Autodesk Inventor part; units mm, degrees
ref_plane "YZ Plane" through (0, 0, 0) normal (1, 0, 0) x (0, 1, 0)
ref_plane "XZ Plane" through (0, 0, 0) normal (0, 1, 0) x (-1, 0, 0)
ref_plane "XY Plane" through (0, 0, 0) normal (0, 0, 1) x (1, 0, 0)
sketch "Skizze1" plane through (0, 0, 0) normal (0, 0, 1) x (1, 0, 0)
  line L0 (-23.5, 19.5) -> (23.5, 19.5)
  line L1 (23.5, 19.5) -> (23.5, -19.5)
  line L2 (23.5, -19.5) -> (-23.5, -19.5)
  line L3 (-23.5, -19.5) -> (-23.5, 19.5)
  line L4 (-23.5, -19.5) -> (23.5, 19.5) construction
  circle A0 centre (-21.0614, 17.0614) radius 1
  circle A1 centre (16, 0) radius 1.5
  line L5 (-23.5, 0) -> (23.5, 0) construction
  circle A2 centre (-21.0614, -17.0614) radius 1
  line L6 (-21.0614, -17.0614) -> (-21.0614, 17.0614) construction
  line L7 (-23.5, 19.5) -> (-21.0614, 17.0614) construction
  line L8 (12.5, -18.5) -> (29.5, -18.5)
  line L9 (29.5, -18.5) -> (29.5, -3.3)
  line L10 (29.5, -3.3) -> (12.5, -3.3)
  line L11 (12.5, -3.3) -> (12.5, -18.5)
  line L12 (12.5, 3.3) -> (29.5, 3.3)
  line L13 (29.5, 3.3) -> (29.5, 18.5)
  line L14 (29.5, 18.5) -> (12.5, 18.5)
  line L15 (12.5, 18.5) -> (12.5, 3.3)
  circle A3 centre (-5.25, -13.5) radius 5
  circle A4 centre (5.25, -13.5) radius 5
  circle A5 centre (-5.25, 13.5) radius 5
  circle A6 centre (5.25, 13.5) radius 5
  circle A7 centre (0, 0) radius 8
  circle A8 centre (0, 0) radius 4
  line L16 (-23.4, 5.9386) -> (-11.75, 5.9386)
  line L17 (-11.75, 5.9386) -> (-11.75, 14.9386)
  line L18 (-11.75, 14.9386) -> (-23.4, 14.9386)
  line L19 (-23.4, 14.9386) -> (-23.4, 5.9386)
  line L20 (-23.4, -15.0614) -> (-16.4, -15.0614)
  line L21 (-16.4, -15.0614) -> (-16.4, 4.9386)
  line L22 (-16.4, 4.9386) -> (-23.4, 4.9386)
  line L23 (-23.4, 4.9386) -> (-23.4, -15.0614)
  line L24 (0, 19.5) -> (0, -19.5) construction
  line L25 (-16.3, -18.5) -> (-10.5, -18.5)
  line L26 (-10.5, -18.5) -> (-10.5, 4.9386)
  line L27 (-10.5, 4.9386) -> (-16.3, 4.9386)
  line L28 (-16.3, 4.9386) -> (-16.3, -18.5)
  dimension "d0" = 39
  dimension "d1" = 47
  dimension "d2" = 3
  dimension "d3" = 2
  dimension "d4" = 38.3
  dimension "d5" = 6
  dimension "d6" = 45
  dimension "d7" = 10
  dimension "d8" = 0.5
  dimension "d9" = 1
  dimension "d10" = 16
  dimension "d11" = 15.2
  dimension "d13" = 6
  dimension "d14" = 17
  dimension "d15" = 15.2
  dimension "d16" = 1
  dimension "d17" = 8
  dimension "d18" = 20
  dimension "d19" = 7
  dimension "d20" = 0.1
  dimension "d21" = 5.8
  dimension "d22" = 0.1
  dimension "d23" = 1
  dimension "d24" = 1
  dimension "d25" = 0.1
  dimension "d26" = 9
  dimension "d27" = 1
  dimension "d28" = 1.5
extrude "Extrusion1" add sketch "Skizze1" against normal blind 2.2 contours L0 L1 L14 L15 L12 L10 L11 L8 L2 L3 | L1 L12 L15 L14 | L8 L11 L10 L1 | A3 | A4 | A5 | A6 | A7 | A8 | L19 L18 L17 L16 | L23 L22 L21 L20 | L28 L27 L26 L25
extrude "Extrusion2" add sketch "Skizze1" along normal blind 16.2 contours L14 L13 L12 L1 | L1 L12 L15 L14 | L8 L11 L10 L1 | L1 L10 L9 L8
sketch "Skizze2" plane through (29.5, -18.5, 0) normal (1, 0, 0) x (0, 0, -1)
  line L0 (-14.8, 1.2) -> (-9.5, 1.2)
  line L1 (-9.5, 1.2) -> (-9.5, 14)
  line L2 (-9.5, 14) -> (-14.8, 14)
  line L3 (-14.8, 14) -> (-14.8, 1.2)
  line L4 (-6.4, 1.2) -> (-1.1, 1.2)
  line L5 (-1.1, 1.2) -> (-1.1, 14)
  line L6 (-1.1, 14) -> (-6.4, 14)
  line L7 (-6.4, 14) -> (-6.4, 1.2)
  line L8 (0, 0) -> (0, 15.2)
  line L9 (-16.2, 15.2) -> (-16.2, 0)
  line L10 (-16.2, 7.6) -> (0, 7.6) construction
  line L11 (0, 38) -> (0, -1)
  point P0 (0, 18.5)
  dimension "d33" = 1.1
  dimension "d34" = 5.3
  dimension "d35" = 5.3
  dimension "d36" = 3.1
  dimension "d37" = 12.8
extrude "Extrusion3" cut sketch "Skizze2" against normal blind 10
extrude "Extrusion4" add sketch "Skizze1" along normal blind 9.5 contours A3 | A4
mirror "Spiegeln1" about plane through (0, 0, 0) normal (0, 1, 0) of "Extrusion4", "Extrusion3"
extrude "Extrusion5" add sketch "Skizze1" along normal blind 13 contours A7
extrude "Extrusion6" add sketch "Skizze1" along normal blind 8 contours L23 L22 L21 L20
extrude "Extrusion11" add sketch "Skizze1" along normal blind 8 contours L19 L18 L17 L16
extrude "Extrusion7" add sketch "Skizze1" along normal blind 7 contours L28 L27 L26 L25
sketch "Skizze3" plane through (-16.3, -18.5, 0) normal (0, -1, 0) x (1, 0, 0)
  line L0 (0, 7) -> (5.8, 7)
  line L1 (0.8004, 7) -> (0.8004, 0.8568)
  line L2 (0.8004, 0.8568) -> (1.6289, 0.8568)
  line L3 (1.6289, 0.8568) -> (1.6289, 7)
  line L4 (2.4575, 7) -> (2.4575, 0.8568)
  line L5 (2.4575, 0.8568) -> (3.2861, 0.8568)
  line L6 (3.2861, 0.8568) -> (3.2861, 7)
  line L7 (4.1146, 7) -> (4.1146, 0.8568)
  line L8 (4.1146, 0.8568) -> (4.9432, 0.8568)
  line L9 (4.9432, 0.8568) -> (4.9432, 7)
  line L10 (0, 0) -> (0, 7)
  line L11 (5.8, 0) -> (5.8, 7)
  point P0 (16.3, 0)
  dimension "d48" = 5.8
  dimension "d49" = 0.8286
  dimension "d50" = 0.8286
  dimension "d51" = 0.8286
extrude "Extrusion8" cut sketch "Skizze3" against normal up to surface (23.4386 mm away)
fillet "Rundung1" radius 0.5 4 edges at (-10.25, -13.5, 9.5) (0.25, -13.5, 9.5) (-10.25, 13.5, 9.5) (0.25, 13.5, 9.5)
sketch "Skizze4" plane through (0, 0, 8) normal (0, 0, 1) x (1, 0, 0)
  circle A0 centre (-19.9, 2.1386) radius 1.6
  circle A1 centre (-19.9, -2.6614) radius 1.6
  circle A2 centre (-19.9, -7.4614) radius 1.6
  circle A3 centre (-19.9, -12.2614) radius 1.6
  line L0 (-16.4, 4.9386) -> (-23.4, 4.9386)
  line L1 (-19.9, 4.9386) -> (-19.9, -15.0614) construction
  line L2 (-16.4, -15.0614) -> (-23.4, -15.0614)
  line L3 (-23.4, -15.0614) -> (-23.4, 4.9386)
  line L4 (-23.4, -5.0614) -> (-16.4, -5.0614) construction
  point P0 (0, 0)
  dimension "d55" = 3.2
  dimension "d56" = 4.8
  dimension "d57" = 4.8
  dimension "d58" = 4.8
extrude "Extrusion9" cut sketch "Skizze4" against normal up to surface (8 mm away)
sketch "Skizze5" plane through (-23.4, -15.0614, 0) normal (-1, 0, 0) x (0, 0, 1)
  line L0 (0.5, 19.15) -> (5, 19.15)
  line L1 (5, 19.15) -> (5, 15.25)
  line L2 (5, 15.25) -> (0.5, 15.25)
  line L3 (0.5, 15.25) -> (0.5, 19.15)
  line L4 (0.5, 14.35) -> (5, 14.35)
  line L5 (5, 14.35) -> (5, 10.45)
  line L6 (5, 10.45) -> (0.5, 10.45)
  line L7 (0.5, 10.45) -> (0.5, 14.35)
  line L8 (0.5, 5.65) -> (5, 5.65)
  line L9 (5, 5.65) -> (5, 9.55)
  line L10 (5, 9.55) -> (0.5, 9.55)
  line L11 (0.5, 9.55) -> (0.5, 5.65)
  line L12 (0.5, 4.75) -> (5, 4.75)
  line L13 (5, 4.75) -> (5, 0.85)
  line L14 (5, 0.85) -> (0.5, 0.85)
  line L15 (0.5, 0.85) -> (0.5, 4.75)
  line L16 (8, 17.2) -> (5, 17.2) construction
  line L17 (0.5, 17.2) -> (5, 17.2) construction
  line L18 (0.5, 12.4) -> (5, 12.4) construction
  line L19 (8, 12.4) -> (5, 12.4) construction
  line L20 (8, 7.6) -> (5, 7.6) construction
  line L21 (0.5, 7.6) -> (5, 7.6) construction
  line L22 (8, 20) -> (8, 0) construction
  line L23 (0.5, 2.8) -> (5, 2.8) construction
  line L24 (5, 2.8) -> (8, 2.8) construction
  line L25 (0, 34.5614) -> (0, -4.4386) construction
  circle A0 centre (4, 25.5) radius 2.5
  line L26 (4, 30) -> (4, 21) construction
  line L27 (8, 25.5) -> (0, 25.5) construction
  line L28 (0, 30) -> (8, 30)
  line L29 (8, 30) -> (8, 21)
  line L30 (0, 21) -> (8, 21)
  line L31 (0, 21) -> (0, 30)
  point P0 (0, 15.0614)
  point P1 (4, 25.5)
  dimension "d61" = 0.5
  dimension "d62" = 4.5
  dimension "d63" = 3.9
  dimension "d66" = 5
extrude "Extrusion10" cut sketch "Skizze5" against normal blind 7 contours L0 L1 L2 L3 | L4 L5 L6 L7 | L11 L10 L9 L8 | L12 L13 L14 L15 | A0
equation "\"d15\" = d11"
properties part number "Step_Down_USB"
Check sheet for the modelled part. Datum: model origin and axes. Units: mm. A direction names the side the tool comes from. Give positions to 0.01 mm unless a question says otherwise; leave off trailing zeros. Write each loop counter-clockwise with the first axis right and the second up, starting at its lowest first coordinate (ties: lowest second). Pieces come first, ordered by that corner, then holes. Notation, with made-up numbers: M 65.5,47.25 L 81.5,47.25 A28 cw 81.5,73.25 Z; hole C 80.25,47 d4. An arc over 180 degrees is marked long. Use one line per item in the form item = value.
(1) Section check C-C on z = 4. State how many separate pieces and enclosed holes the cut face has, plus the area to 3 significant figures.
Answer block:
separate_pieces = 17
enclosed_holes = 1
area = 904 mm2
(2) Section check B-B on x = 16. Record the boundary of the cut face in (y, z).
Answer block:
outline = M -19.5,-2.2 L -1.5,-2.2 L -1.5,0 L -3.3,0 L -3.3,16.2 L -18.5,16.2 L -18.5,0 L -19.5,0 Z; M 1.5,-2.2 L 19.5,-2.2 L 19.5,0 L 18.5,0 L 18.5,16.2 L 3.3,16.2 L 3.3,0 L 1.5,0 Z
(3) Draft check along Y on faces 1 (the flat face through (-15.5, -7, 4)), 2 (the cylindrical face through (-21.08, -6.38, 6.52)), 3 (the flat face through (21, 18.5, 8)). Enter one of: pulls with the +Y half, pulls with the -Y half, needs draft (parallel to the pull), parting line crosses it, or undercut.
Answer block:
face_1 = needs draft
face_2 = undercut
face_3 = pulls with the +Y half
(4) Section check A-A on z = 11.5. Record the boundary of the cut face in (x, y).
Answer block:
outline = C 0,0 d16; M 12.5,-18.5 L 29.5,-18.5 L 29.5,-17.3 L 19.5,-17.3 L 19.5,-4.5 L 29.5,-4.5 L 29.5,-3.3 L 12.5,-3.3 Z; M 12.5,3.3 L 29.5,3.3 L 29.5,4.5 L 19.5,4.5 L 19.5,17.3 L 29.5,17.3 L 29.5,18.5 L 12.5,18.5 Z; hole C 0,0 d8
(5) Depth check by flat-ended pin: P1, Ø4.5, axis at x = -12.5, z = 5, coming from the +Y side; P2, Ø1.3, axis at x = -21.5, z = 3.5, coming from the -Y side; P3, Ø1, axis at y = -1, z = 5, coming from the -X side; P4, Ø6.5, axis at x = -14.5, z = 2.5, coming from the -Y side. Enter the tip coordinate at first touch or a pass-through.
Answer block:
P1 = 14.94
P2 = -15.06
P3 = -23.4
P4 = -19.5
(6) Tool access check on faces 4 (the flat face through (21, 3.3, 8)), 5 (the cylindrical face through (-21.08, -11.18, 6.52)), 6 (the flat face through (-22, 2, 0.5)), 7 (the flat face through (25, 4.5, 12)). Record the directions out of +Z, -Z, +X, -X, +Y, -Y that give a thin tool (end or side, any length) a straight path to the whole face; none if there is none.
Answer block:
face_4 = +Z, +X
face_5 = +Z
face_6 = -X
face_7 = +X
(7) Material ranges on line 1 along Y through (x, z) = (-19.9, 0.3); line 2 along Y through (x, z) = (25, 5.5); line 3 along Y through (x, z) = (3, 1.5), recorded low to high.
Answer block:
line_1 = -15.06 to -13.86, -10.66 to -9.06, -5.86 to -4.26, -1.06 to 0.54, 3.74 to 4.94, 5.94 to 14.94
line_2 = -18.5 to -17.3, -4.5 to -3.3, 3.3 to 4.5, 17.3 to 18.5
line_3 = -17.97 to -9.03, -7.42 to -2.65, 2.65 to 7.42, 9.03 to 17.97
